Geometry: final body of the model. Coordinates: model frame, mm. A direction names the side the tool comes from. Give positions to 0.01 mm unless a question says otherwise; leave off trailing zeros. Loops run counter-clockwise (first coordinate to the right, second up) from the corner with the lowest first, then second, coordinate; pieces in that order, holes last. Notation, with made-up numbers: (27.5, -0.5) - (65.5, -0.5) arc R12 cw to (65.5, 17.5) - close; hole circle Ø10 at (-8.5, -30.75). An arc over 180 degrees is marked (long way). Answer in a Markdown table with one row per item.
from build123d import *

# Parameters (mm, degrees)
SKETCH2_R                                        = 50.8
FLANGE_DEPTH                                     = 12.7
SKETCH3_R                                        = 25.4
HUB_DEPTH                                        = 25.4
SKETCH4_R                                        = 12.7
BORE_DEPTH                                       = 82.319677815
CBORE_FOR_1_4_SOCKET_HEAD_CAP_SCREW2_D           = 7.112
CBORE_FOR_1_4_SOCKET_HEAD_CAP_SCREW2_CBORE_D     = 11.176
CBORE_FOR_1_4_SOCKET_HEAD_CAP_SCREW2_CBORE_DEPTH = 6.35


with BuildPart() as part:
    # Sketch2 → Flange (new body)
    with BuildSketch(Plane(origin=(0, 0, 0), x_dir=(1, 0, 0), z_dir=(0, 1, 0))):
        with Locations(Location((0, 0, 0), (0, 0, 270))):
            Circle(SKETCH2_R)
    extrude(amount=FLANGE_DEPTH)

    # Sketch3 → Hub (add)
    with BuildSketch(Plane(origin=(0, 12.7, 0), x_dir=(1, 0, 0), z_dir=(0, 1, 0))):
        with Locations(Location((0, 0, 0), (0, 0, 270))):
            Circle(SKETCH3_R)
    extrude(amount=HUB_DEPTH)

    # Sketch4 → Bore (cut, through all)
    with BuildSketch(Plane(origin=(0, 38.1, 0), x_dir=(1, 0, 0), z_dir=(0, 1, 0))):
        with Locations(Location((0, 0, 0), (0, 0, 270))):
            Circle(SKETCH4_R)
    extrude(amount=-BORE_DEPTH, mode=Mode.SUBTRACT)

    # CBORE for 1/4 Socket Head Cap Screw2 (through all)
    with Locations(Plane(origin=(0, 12.7, 0), x_dir=(1, 0, 0), z_dir=(0, 1, 0))):
        with Locations((38.1, 0)):
            CounterBoreHole(CBORE_FOR_1_4_SOCKET_HEAD_CAP_SCREW2_D / 2, CBORE_FOR_1_4_SOCKET_HEAD_CAP_SCREW2_CBORE_D / 2, CBORE_FOR_1_4_SOCKET_HEAD_CAP_SCREW2_CBORE_DEPTH)


solid = part.part
Q1. Draft query along X for faces 3 (the flat face through (12, 38.1, 5)), 4 (the cylindrical face through (-30.911, 6.261, -40.313)), 5 (the cylindrical face through (41.653, 3.131, -0.156)). Return one class per face: pulls with the +X half, pulls with the -X half, needs draft (parallel to the pull), parting line crosses it, or undercut.
Check values:
| item | result |
|---|---|
| face 3 | needs draft |
| face 4 | parting line crosses it |
| face 5 | undercut |
Q2. Cut plane C-C (x = 15.5). Output: boundary loops of the cut face in (y, z).
Check values:
| item | result |
|---|---|
| outline | (0, -48.38) - (12.7, -48.38) - (12.7, -20.12) - (38.1, -20.12) - (38.1, 20.12) - (12.7, 20.12) - (12.7, 48.38) - (0, 48.38) - close |
Q3. Reachability of faces 1 (the cylindrical face through (-7.7, 19.3, -10.1)), 2 (the cylindrical face through (43.43, 9.57, -1.68)) from +Z, -Z, +X, -X, +Y, -Y: full face, straight path, thin tool, end or side. Return the list, or none.
Check values:
| item | result |
|---|---|
| face 1 | +Y, -Y |
| face 2 | +Y |
Q4. Cut plane A-A (z = 0). Output: boundary loops of the cut face in (x, y).
Check values:
| item | result |
|---|---|
| outline | (-50.8, 0) - (-12.7, 0) - (-12.7, 38.1) - (-25.4, 38.1) - (-25.4, 12.7) - (-50.8, 12.7) - close; (12.7, 0) - (34.54, 0) - (34.54, 6.35) - (32.51, 6.35) - (32.51, 12.7) - (25.4, 12.7) - (25.4, 38.1) - (12.7, 38.1) - close; (41.66, 0) - (50.8, 0) - (50.8, 12.7) - (43.69, 12.7) - (43.69, 6.35) - (41.66, 6.35) - close |
Q5. Cut plane D-D (y = 25). Output: boundary loops of the cut face in (x, z), and give its area (3 significant figures).
Check values:
| item | result |
|---|---|
| outline | circle Ø50.8 at (0, 0); hole circle Ø25.4 at (0, 0) |
| area | 1,520 mm² |
Q6. Cut plane B-B (x = 0). Output: boundary loops of the cut face in (y, z), and give its area (3 significant figures).
Check values:
| item | result |
|---|---|
| outline | (0, -50.8) - (12.7, -50.8) - (12.7, -25.4) - (38.1, -25.4) - (38.1, -12.7) - (0, -12.7) - close; (0, 12.7) - (38.1, 12.7) - (38.1, 25.4) - (12.7, 25.4) - (12.7, 50.8) - (0, 50.8) - close |
| area | 1,610 mm² |
Q7. First-contact query: pin 1 (5 mm diameter, centred on x = -14.5, y = 18, fed in from -Z); pin 2 (6 mm diameter, centred on y = 12, z = 23, fed in from +X); pin 3 (1 mm diameter, centred on x = -37, y = 7, fed in from -Z). Flat tips, straight axial feed; report the tip coordinate or a pass-through.
Check values:
| item | result |
|---|---|
| pin 1 | z = -22.39 |
| pin 2 | x = 46.7 |
| pin 3 | z = -35.33 |
Q8. Material intervals for line 1 along Y through (x, z) = (30.5, 39); line 2 along X through (y, z) = (19.5, -9); line 3 along Z through (x, y) = (38.1, 8.25), sorted ascending.
Check values:
| item | result |
|---|---|
| line 1 | 0 to 12.7 |
| line 2 | -23.75 to -8.96, 8.96 to 23.75 |
| line 3 | -33.6 to -5.59, 5.59 to 33.6 |
